Geometry check sheet. Reference: the model listing, model coordinates, mm. Face numbers are marked on the shaded views. A direction names the side the tool comes from. Coordinates: 2 decimals unless noted, no trailing zeros. Write each loop counter-clockwise with the first axis right and the second up, starting at its lowest first coordinate (ties: lowest second). Pieces come first, ordered by that corner, then holes. Notation, with made-up numbers: (-16.5, 37.5) -> (5.5, 37.5) arc R28 cw to (5.5, 55.5) -> close; hole circle Ø11 at (6, -32.75). An arc over 180 degrees is marked (long way). Answer as CSV lines item,"result".
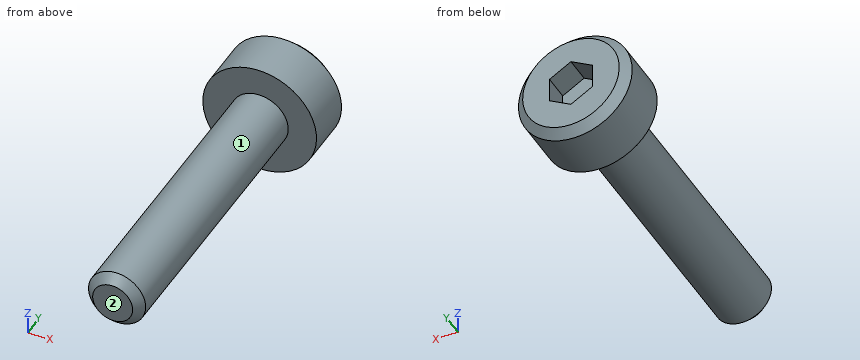
```python
from build123d import *

# Parameters (mm, degrees)
CUT_EXTRUDE1_DEPTH = 0.9


with BuildPart() as part:
    # Sketch1 → Revolve1 (revolve)
    with BuildSketch(Plane.XY, mode=Mode.PRIVATE) as revolve1_sk:
        Polygon((0, -10), (0.7, -10), (1, -9.7), (1, 0), (1.99, 0), (1.99, 1.7), (1.69, 2), (0, 2), align=None)
    revolve(revolve1_sk.sketch.rotate(Axis((0, -10, 0), (0, 1, 0)), 90), axis=Axis((0, -10, 0), (0, 1, 0)))

    # Sketch2 → Cut-Extrude1 (cut)
    with BuildSketch(Plane(origin=(0, 2, 0), x_dir=(1, 0, 0), z_dir=(0, 1, 0))):
        Polygon((0.75, -0.433012702), (0, -0.866025404), (-0.75, -0.433012702), (-0.75, 0.433012702), (0, 0.866025404), (0.75, 0.433012702), align=None)
    extrude(amount=-CUT_EXTRUDE1_DEPTH, mode=Mode.SUBTRACT)


solid = part.part
```
Item 1: Depth check by flat-ended pin: pin 1 Ø0.5 at (x, z) = (0, 0.5) entering from +Y; pin 2 Ø1 at (x, y) = (-1.5, 0) entering from -Z. Enter the tip coordinate at first touch or a pass-through.
Responses:
pin 1,"stops at y = 1.1"
pin 2,"stops at z = -1.72"
Item 2: Thickness scan on probe 1 along X at (y, z) = (-4.5, -0.5); probe 2 along Y at (x, z) = (0.15, 1.5); probe 3 along Y at (x, z) = (0.1, -0.3). Record the ranges inside material, lowest first.
Responses:
probe 1,"x = -0.87 to 0.87"
probe 2,"y = 0 to 2"
probe 3,"y = -10 to 1.1"
Item 3: Cross-section at A-A, the plane z = 0. Record the cut outline in (x, y), plus the area to 3 significant figures.
Responses:
outline,"(-1.99, 0) -> (-1, 0) -> (-1, -9.7) -> (-0.7, -10) -> (0.7, -10) -> (1, -9.7) -> (1, 0) -> (1.99, 0) -> (1.99, 1.7) -> (1.69, 2) -> (0.75, 2) -> (0.75, 1.1) -> (-0.75, 1.1) -> (-0.75, 2) -> (-1.69, 2) -> (-1.99, 1.7) -> close"
area,"26.4 mm2"
Item 4: Set-up check for the marked faces 1 and 2: record each of +Z, -Z, +X, -X, +Y, -Y from which the full face is reachable in a straight line by a thin tool's end or side.
Responses:
face 1,"-Y"
face 2,"+Z, -Z, +X, -X, -Y"
Item 5: Cross-section at B-B, the plane y = -9. Record the cut outline in (x, z), plus the area to 3 significant figures.
Responses:
outline,"circle Ø2 at (0, 0)"
area,"3.14 mm2"
